For this review, use the dimensioned drawing (mm, ordinates from the lowest corner) and the shaded views. Round coordinates to 2 decimals unless told otherwise and drop trailing zeros. Order: outer loops, then holes, each group sorted by start corner. A loop starts at its lowest first (then second) coordinate and runs counter-clockwise, first axis right, second up. Notation, with made-up numbers: (68, 66.25) -> (113, 66.25) arc R20 ccw to (113, 84.25) -> close; hole circle Ø3 at (39.5, 84.25). An arc over 180 degrees is marked (long way). Answer in a Markdown table with one row per item.
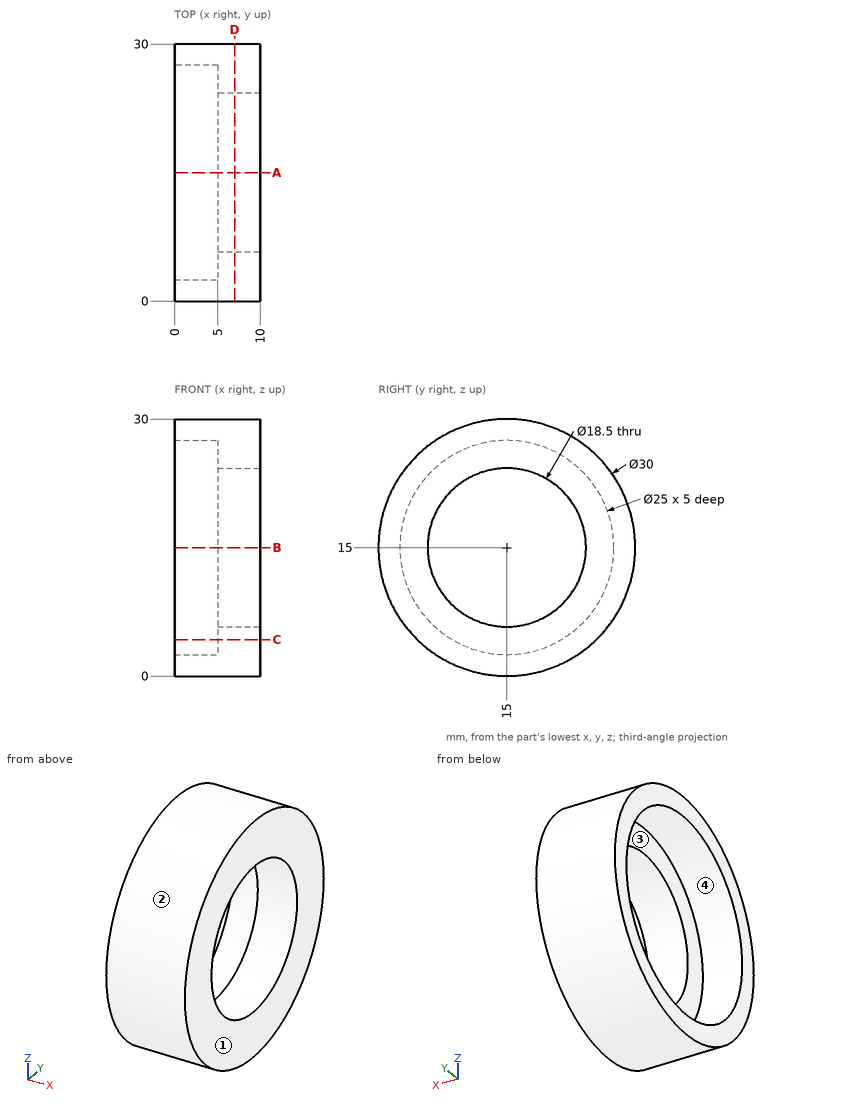
Q1. Take a section at C-C, the plane z = 4.25. Write out the cut boundary in (x, y).
Answer key:
| item | result |
|---|---|
| outline | (0, 4.54) -> (10, 4.54) -> (10, 25.46) -> (0, 25.46) -> (0, 21.38) -> (5, 21.38) -> (5, 8.62) -> (0, 8.62) -> close |
Q2. To check wall thickness, follow probe 1 along Z at (x, y) = (2.6, 15); probe 2 along Z at (x, y) = (7.9, 15); probe 3 along X at (y, z) = (25.5, 20). State the ranges of each line that lie inside material, in increasing order.
Answer key:
| item | result |
|---|---|
| probe 1 | z = 0 to 2.5, 27.5 to 30 |
| probe 2 | z = 0 to 5.75, 24.25 to 30 |
| probe 3 | x = 5 to 10 |
Q3. The part is to be moulded in two halves that separate along Y. For the marked faces 1, 2, 3 and 4, say which applies: +Y half, -Y half, draft (parallel to the pull), parting line (faces both ways), or undercut.
Answer key:
| item | result |
|---|---|
| face 1 | draft |
| face 2 | parting line |
| face 3 | undercut |
| face 4 | undercut |
Q4. Take a section at D-D, the plane x = 7. Write out the cut boundary in (y, z).
Answer key:
| item | result |
|---|---|
| outline | circle Ø30 at (15, 15); hole circle Ø18.5 at (15, 15) |
Q5. Take a section at A-A, the plane y = 15. Write out the cut boundary in (x, z).
Answer key:
| item | result |
|---|---|
| outline | (0, 0) -> (10, 0) -> (10, 5.75) -> (5, 5.75) -> (5, 2.5) -> (0, 2.5) -> close; (0, 27.5) -> (5, 27.5) -> (5, 24.25) -> (10, 24.25) -> (10, 30) -> (0, 30) -> close |
Q6. Clearance check with flat-ended pins moving along their axes: pin 1 Ø1.5 at (x, y) = (1.5, 19.5) entering from -Z; pin 2 Ø1.5 at (y, z) = (17, 8) entering from -X; pin 3 Ø4 at (y, z) = (20, 21) entering from -X. State where each tip first meets the part, or that it passes through.
Answer key:
| item | result |
|---|---|
| pin 1 | stops at z = 0.48 |
| pin 2 | passes through |
| pin 3 | stops at x = 5 |
